Autodesk Inventor part; units mm, degrees
ref_plane "YZ Plane" through (0, 0, 0) normal (1, 0, 0) x (0, 1, 0)
ref_plane "XZ Plane" through (0, 0, 0) normal (0, 1, 0) x (-1, 0, 0)
ref_plane "XY Plane" through (0, 0, 0) normal (0, 0, 1) x (1, 0, 0)
sketch "Sketch1" plane through (0, 0, 0) normal (0, 1, 0) x (-1, 0, 0)
  line L0 (-75, 55) -> (75, 55)
  line L1 (75, 55) -> (75, -55)
  line L2 (75, -55) -> (-75, -55)
  line L3 (-75, -55) -> (-75, 55)
  line L4 (-75, 55) -> (75, -55) construction
  line L5 (75, 55) -> (-75, -55) construction
  point P0 (0, 0)
  dimension "d0" = 150
  dimension "d1" = 110
extrude "Extrusion1" add sketch "Sketch1" along normal blind 7
sketch "Sketch9" plane through (0, 7, 0) normal (0, 1, 0) x (1, 0, 0)
  line L0 (-75, 55) -> (-75, -55) construction
  line L1 (-75, -55) -> (75, -55) construction
  line L2 (-62, 57.15) -> (-62, -57.15) construction
  line L3 (75, 55) -> (-75, 55) construction
  line L4 (75, 55) -> (-75, 55) construction
  line L5 (75, -55) -> (75, 55) construction
  line L6 (62, -57.15) -> (62, 57.15) construction
  line L7 (-75, -55) -> (75, -55) construction
  line L8 (-75, -57.15) -> (-62, -57.15) construction
  line L9 (-69.1, 0) -> (-69.1, -25.4) construction
  line L10 (-69.1, 0) -> (-69.1, 25.4) construction
  circle A0 centre (-69.1, 25.4) radius 3.365
  circle A1 centre (-69.1, -25.4) radius 3.365
  point P0 (0, 0)
  point P1 (54, 57.15)
  point P2 (54, -57.15)
  point P3 (-54, -57.15)
  point P4 (-54, 57.15)
  dimension "d36" = 25.4
  dimension "d37" = 25.4
  dimension "d38" = 6.73
  dimension "d39" = 6.73
extrude "Extrusion9" cut sketch "Sketch9" against normal blind 10
ref_plane "Work Plane2" through (-1.2, 0, 55) normal (1, 0, 0) x (0, 0, -1)
mirror "Mirror2" about plane through (-1.2, 0, 55) normal (1, 0, 0) of "Extrusion9"
properties part number "cooling plate"
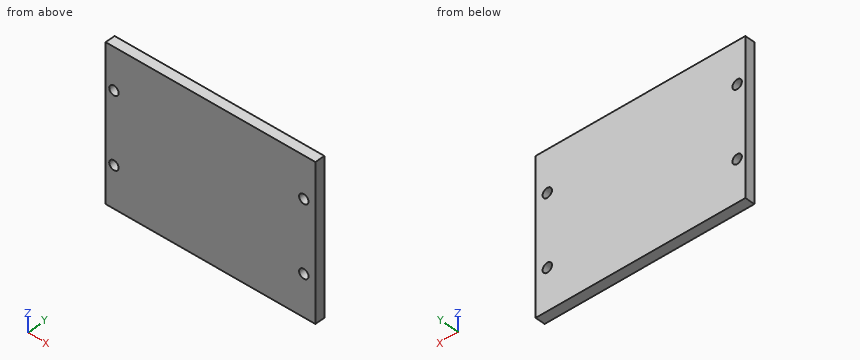
CAD build for the part. Positions are in the model's coordinates, mm. Coordinates: 2 decimals unless noted, no trailing zeros. Write each loop counter-clockwise with the first axis right and the second up, starting at its lowest first coordinate (ties: lowest second). Pieces come first, ordered by that corner, then holes. Notation, with made-up numbers: (31.5, 63) - (52.5, 63) arc R15 cw to (52.5, 88) - close; hole circle Ø3 at (-34.75, 19.5). An arc over 180 degrees is marked (long way). Use a Markdown table: item, result. Add a question column.
Item 1: Band-saw the part on A-A, the plane z = -25.4. Give the cut face in (x, y) (3 decimals).
Item 2: Band-saw the part on B-B, the plane x = -69.1. Give the cut face in (y, z) (3 decimals), and give its area (3 significant figures).
Item 3: Drill centre lines: L1, parallel to Z at x = -69.1, y = 5.25 (3 decimals); L2, parallel to X at y = 2.75, z = -25.4 (3 decimals); L3, parallel to X at y = 5.75, z = 27. Where is each one in solid material? Low to high. Write a range as from..to.
Item 4: Flat gauge pin, fed straight in: pin 1 (5.5 mm diameter, centred on x = 66.7, z = 25.4, fed in from +Y). Where does the tip first touch, or does it go through?
Numbers:
| question | item | result |
|---|---|---|
| 1 | outline | (-75, 0) - (-72.465, 0) - (-72.465, 7) - (-75, 7) - close; (-65.735, 0) - (63.335, 0) - (63.335, 7) - (-65.735, 7) - close; (70.065, 0) - (75, 0) - (75, 7) - (70.065, 7) - close |
| 2 | outline | (0, -55) - (7, -55) - (7, -28.765) - (0, -28.765) - close; (0, -22.035) - (7, -22.035) - (7, 22.035) - (0, 22.035) - close; (0, 28.765) - (7, 28.765) - (7, 55) - (0, 55) - close |
| 2 | area | 676 mm2 |
| 3 | L1 | -55..-28.765, -22.035..22.035, 28.765..55 |
| 3 | L2 | -75..-72.465, -65.735..63.335, 70.065..75 |
| 3 | L3 | -75..-72.06, -66.14..63.74, 69.66..75 |
| 4 | pin 1 | through |
